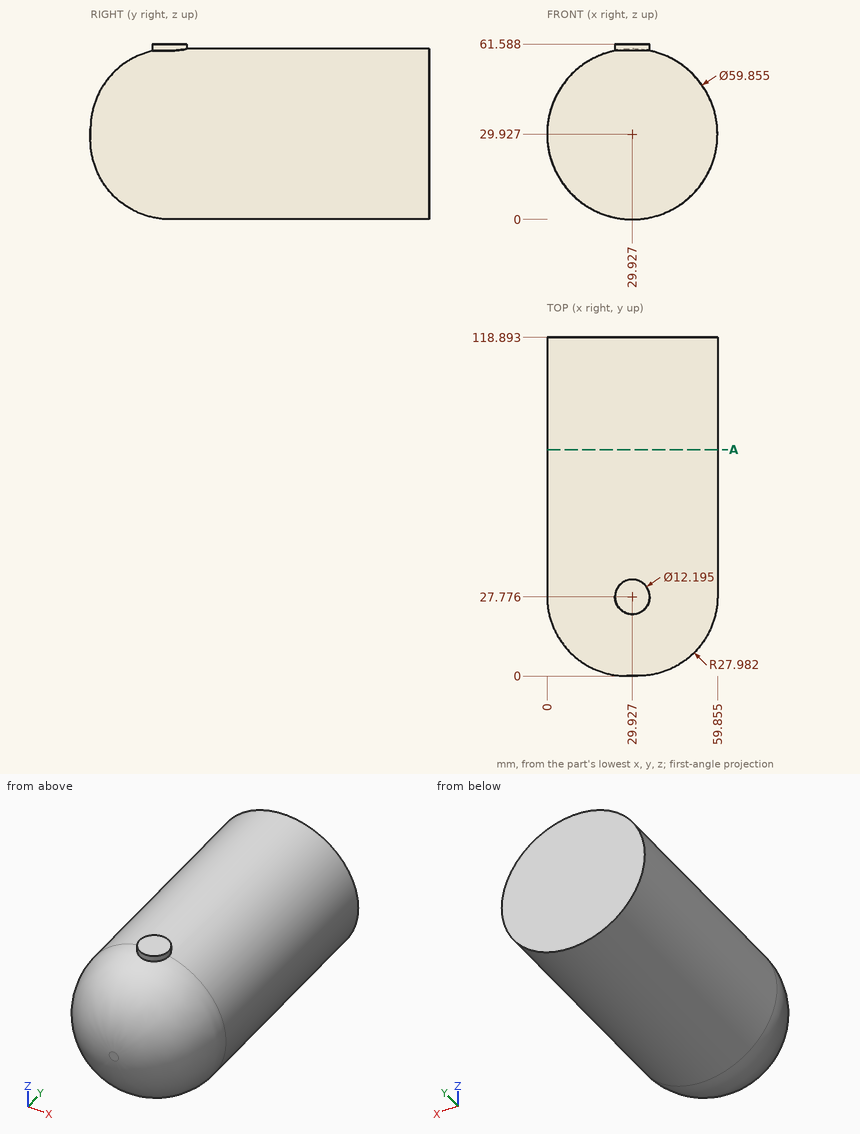
For this review, use the dimensioned drawing (mm, ordinates from the lowest corner) and the shaded views. Give positions to 0.01 mm unless a question says otherwise; leave off trailing zeros. Order: outer loops, then holes, each group sorted by start corner. A loop starts at its lowest first (then second) coordinate and runs counter-clockwise, first axis right, second up. Notation, with made-up numbers: (58.5, -30.5) - (100.5, -30.5) arc R23 cw to (100.5, -17.5) - close; hole circle Ø7 at (65.5, 53). An arc over 180 degrees is marked (long way). Write item = value, one per line. Start each with the question number.
Q1. Clearance check with flat-ended pins moving along their axes: pin 1 Ø6 at (y, z) = (73.5, 19) entering from -X; pin 2 Ø12 at (y, z) = (45.5, 12.5) entering from -X; pin 3 Ø2 at (x, z) = (54, 26) entering from -Y. State where each tip first meets the part, or that it passes through.
Q2. To check wall thickness, follow L1, parallel to X at y = 14.5, z = 42 (1 decimal); L2, parallel to X at y = 91.5, z = 26.5; L3, parallel to Y at x = 36, z = 17 (1 decimal). State the ranges of each line that lie inside material, in increasing order. Write a range as from..to.
Q3. We need section A-A on y = 79.5. State the section outline as (x, z) points (1 decimal), plus the area to 3 significant figures.
Working result:
q1.pin_1 = 1.07
q1.pin_2 = 2.27
q1.pin_3 = 10.01
q2.L1 = 6.4..53.5
q2.L2 = 0.2..59.66
q2.L3 = 2.9..118.9
q3.outline = circle Ø59.9 at (29.9, 29.9)
q3.area = 2,810 mm²
